Read the model definition and answer for the solid it produces. Units are mm, in the model's axes. A direction names the side the tool comes from. Coordinates: 2 decimals unless noted, no trailing zeros. Loops run counter-clockwise (first coordinate to the right, second up) from the corner with the lowest first, then second, coordinate; pieces in that order, holes last. Notation, with made-up numbers: (5, 68) -> (41, 68) arc R8 cw to (41, 76) -> close; hole circle Ø4 at (-10.5, 51). An arc over 180 degrees is marked (long way). Answer as a JSON object with one key per item and string values. Group by question number.
1) Consider probe 1 along X at (y, z) = (-1, 10); probe 2 along Y at (x, z) = (0, 17.25); probe 3 along Y at (x, z) = (0, -0.85). Determine where each line is inside the solid, lowest interval first. Write a range as [from, to].
2) Flat-ended cylindrical pins translate along their axes: P1, Ø8, axis at x = -13, z = 6, coming from the -Y side; P2, Ø3, axis at y = 47.5, z = 15.5, coming from the +X side; P3, Ø10, axis at x = -25, z = 7, coming from the +Y side. Find the tip coordinate at first contact, or state that the pin passes through.
3) Which of the six approach directions +Z, -Z, +X, -X, +Y, -Y give full straight-line access (tool end or side, diameter ignored) to faces 1 (the face through (-52.3, -64.4, 21.8)), 2 (the face through (67.453, -51.721, -0.986))?
4) Section A-A, the plane x = 0 is taken. Give the vertices of the cut face in (y, z), plus the area to 3 significant figures.
5) Section C-C, the plane z = 16.75 is taken. Give the vertices of the cut face in (x, y), plus the area to 3 significant figures.
from build123d import *

# Parameters (mm, degrees)
SKETCH1_R                       = 87.5
SKETCH1_R_2                     = 83.75
BOSS_EXTRUDE1_DEPTH             = 21.8
SKETCH2_R                       = 85
SKETCH2_R_2                     = 82.75
BOSS_EXTRUDE2_DEPTH             = 2
BOSS_EXTRUDE2_DIRECTION_2_REACH = 127.649


with BuildPart() as part:
    # Sketch1 → Boss-Extrude1 (new body)
    with BuildSketch(Plane.XY):
        Circle(SKETCH1_R)
        Circle(SKETCH1_R_2, mode=Mode.SUBTRACT)
    extrude(amount=BOSS_EXTRUDE1_DEPTH)

    # Sketch2 → Boss-Extrude2 (add)
    with BuildSketch(Plane(origin=(0, 0, 0), x_dir=(-1, 0, 0), z_dir=(0, 0, -1))):
        Circle(SKETCH2_R)
        Circle(SKETCH2_R_2, mode=Mode.SUBTRACT)
    extrude(amount=BOSS_EXTRUDE2_DEPTH)

    # Boss-Extrude2 direction 2: up to this face of the body (flat: up to its plane)
    boss_extrude2_direction_2_end = Plane(part.part.faces().sort_by_distance((-85.025126266, 0, 21.8))[0])
    # Sketch2 → Boss-Extrude2 direction 2 (add, up to the picked face)
    with BuildSketch(Plane(origin=(0, 0, 0), x_dir=(-1, 0, 0), z_dir=(0, 0, -1)), mode=Mode.PRIVATE) as boss_extrude2_direction_2_sk1:
        Circle(SKETCH2_R)
        Circle(SKETCH2_R_2, mode=Mode.SUBTRACT)
    boss_extrude2_direction_2_tool1 = split(extrude(boss_extrude2_direction_2_sk1.sketch, amount=-BOSS_EXTRUDE2_DIRECTION_2_REACH, mode=Mode.PRIVATE), bisect_by=boss_extrude2_direction_2_end, keep=Keep.BOTH, mode=Mode.PRIVATE)
    add(boss_extrude2_direction_2_tool1.solids().sort_by(Axis((84.759584, 0, 0), (0, 0, 1)))[0])


solid = part.part
Determined:
{
 "1": {"probe 1": "[-87.49, -82.74], [82.74, 87.49]", "probe 2": "[-87.5, -82.75], [82.75, 87.5]", "probe 3": "[-85, -82.75], [82.75, 85]"},
 "2": {"P1": "y = -87.04", "P2": "x = 74.43", "P3": "y = 85.18"},
 "3": {"face 1": "+Z, +X, -X, +Y, -Y", "face 2": "-Z"},
 "4": {"outline": "(-87.5, 0) -> (-85, 0) -> (-85, -2) -> (-82.75, -2) -> (-82.75, 21.8) -> (-87.5, 21.8) -> close; (82.75, -2) -> (85, -2) -> (85, 0) -> (87.5, 0) -> (87.5, 21.8) -> (82.75, 21.8) -> close", "area": "216 mm²"},
 "5": {"outline": "circle Ø175 at (0, 0); hole circle Ø165.5 at (0, 0)", "area": "2,540 mm²"}
}
